```python
from build123d import *

# Parameters (mm, degrees)
EXTRUDE_1_DEPTH          = 22.5
EXTRUDE_2_DEPTH          = 5
EXTRUDE_3_DEPTH          = 4
CUT_EXTRUDE_1_DEPTH      = 23
CUT_EXTRUDE_1_DEPTH_BACK = 8
SKETCH_2_4_R             = 4
CUT_EXTRUDE_2_DEPTH      = 17.5
FILLET_1_R               = 5
SKETCH_4_R               = 4
CUT_EXTRUDE_4_DEPTH      = 35
SKETCH_5_R               = 4
CUT_EXTRUDE_5_DEPTH      = 47
FILLET_2_R               = 10
FILLET_3_R               = 1
CHAMFER_1_SIZE           = 1.6


with BuildPart() as part:
    # Sketch 1 → Extrude 1 (new, symmetric)
    with BuildSketch(Plane.XY):
        Polygon((0, 0), (135, 0), (135, 8), (107, 8), (107, 40), (57, 40), (32, 8), (0, 8), align=None)
    extrude(amount=EXTRUDE_1_DEPTH, both=True)

    # Sketch 2 → Extrude 2 (add, symmetric)
    with BuildSketch(Plane.XY):
        with BuildLine():
            Line((8, 8), (8, 25))
            ThreePointArc((8, 25), (10.343145751, 30.656854249), (16, 33))
            Line((16, 33), (51.53125, 33))
            Line((51.53125, 33), (32, 8))
            Line((32, 8), (8, 8))
        make_face()
    extrude(amount=EXTRUDE_2_DEPTH, both=True)

    # Sketch 2_3 → Extrude 3 (add, symmetric)
    with BuildSketch(Plane.XY):
        Polygon((107, 40), (135, 8), (107, 8), align=None)
    extrude(amount=EXTRUDE_3_DEPTH, both=True)

    # Sketch 2_4 → Cut-Extrude 1 (cut, two sides: drawn at the far end of the back side and taken through both)
    with BuildSketch(Plane.XY.offset(-CUT_EXTRUDE_1_DEPTH_BACK)):
        with Locations((16, 25)):
            Circle(SKETCH_2_4_R)
    extrude(amount=CUT_EXTRUDE_1_DEPTH + CUT_EXTRUDE_1_DEPTH_BACK, mode=Mode.SUBTRACT)

    # Sketch 3 → Cut-Extrude 2 (cut, symmetric)
    with BuildSketch(Plane.XY):
        Polygon((35.901970252, 0), (59.339470252, 30), (91, 30), (91, 0), align=None)
    extrude(amount=CUT_EXTRUDE_2_DEPTH, both=True, mode=Mode.SUBTRACT)

    # Fillet 1
    fillet_1_edges = [part.edges().sort_by_distance(p)[0] for p in [
        (107, 8, 13.25),
        (107, 8, -13.25),
    ]]
    fillet(fillet_1_edges, radius=FILLET_1_R)

    # Sketch 4 → Cut-Extrude 4 (cut)
    with BuildSketch(Plane.XZ):
        with Locations(Location((7.5, 15, 0), (0, 0, 270))):
            Circle(SKETCH_4_R)
        with Locations((7.5, -15)):
            Circle(SKETCH_4_R)
        with Locations((127.5, -15)):
            Circle(SKETCH_4_R)
        with Locations(Location((127.5, 15, 0), (0, 0, 270))):
            Circle(SKETCH_4_R)
    extrude(amount=-CUT_EXTRUDE_4_DEPTH, mode=Mode.SUBTRACT)

    # Sketch 5 → Cut-Extrude 5 (cut)
    with BuildSketch(Plane(origin=(0, 40, 0), x_dir=(1, 0, 0), z_dir=(0, 1, 0))):
        with Locations(Location((98, 0, 0), (0, 0, 180))):
            Circle(SKETCH_5_R)
    extrude(amount=-CUT_EXTRUDE_5_DEPTH, mode=Mode.SUBTRACT)

    # Fillet 2
    fillet_2_edges = [part.edges().sort_by_distance(p)[0] for p in [
        (135, 4, 22.5),
        (0, 4, -22.5),
        (0, 4, 22.5),
        (135, 4, -22.5),
    ]]
    fillet(fillet_2_edges, radius=FILLET_2_R)

    # Fillet 3
    fillet_3_edges = [part.edges().sort_by_distance(p)[0] for p in [
        (41.765625, 20.5, 5),
        (41.765625, 20.5, -5),
        (91, 15, -17.5),
        (91, 30, 0),
        (47.620720252, 15, -17.5),
        (75.169735126, 30, -17.5),
        (59.339470252, 30, 0),
        (91, 15, 17.5),
        (75.169735126, 30, 17.5),
        (47.620720252, 15, 17.5),
    ]]
    fillet(fillet_3_edges, radius=FILLET_3_R)

    # Chamfer 1
    chamfer_1_edges = [part.edges().sort_by_distance(p)[0] for p in [
        (102, 40, 0),
    ]]
    chamfer(chamfer_1_edges, length=CHAMFER_1_SIZE)


solid = part.part
```
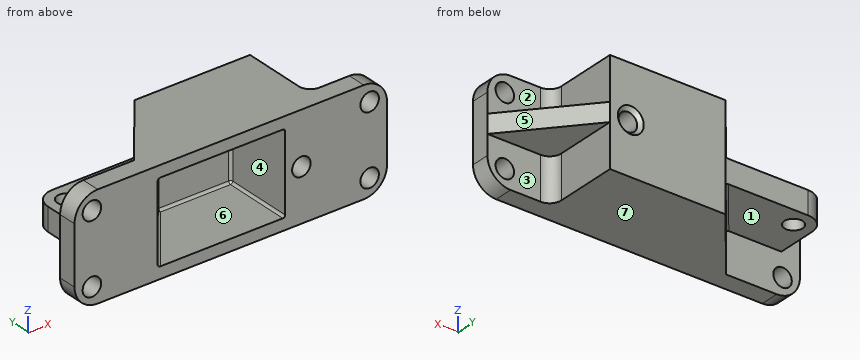
Can you work these out from the model? Positions are in its coordinate system, mm. Face numbers are marked on the shaded views. A direction names the side the tool comes from. Give positions to 0.01 mm unless a question says otherwise; leave off trailing zeros. Loops run counter-clockwise (first coordinate to the right, second up) from the corner with the lowest first, then second, coordinate; pieces in that order, holes last. Notation, with made-up numbers: M 59,18.25 L 118,18.25 A24 cw 118,56.25 Z; hole C 4.5,43 d5. An arc over 180 degrees is marked long. One line per item, written item: value.
(1) I need wall thicknesses on line 1 (Z direction, x = 56.5, y = 24); line 2 (X direction, y = 3, z = 15); line 3 (X direction, y = 25, z = -1) (3 decimals). Which ranges of each line are inside material? Lowest first, please.
Returned:
line 1: -22.5 to -17.5, 17.5 to 22.5
line 2: 0.32 to 3.5, 11.5 to 38.25, 91 to 123.5, 131.5 to 134.68
line 3: 8 to 12, 20 to 55.433, 91 to 94.127, 101.873 to 120.125
(2) Suppose I cut it at A-A on z = 0. List the corners of the cut face in (x, y) for me.
Returned:
outline: M 0,0 L 35.9,0 L 59.04,29.62 A1 cw 59.83,30 L 90,30 A1 cw 91,29 L 91,0 L 94,0 L 94,38.4 L 92.4,40 L 57,40 L 51.53,33 L 16,33 A8 ccw 8,25 L 8,8 L 0,8 Z; M 102,0 L 135,0 L 135,8 L 107,40 L 103.6,40 L 102,38.4 Z; hole C 16,25 d8
(3) Will these pins go through, and if not, where does the flat tip stop? pin 1 (15 mm diameter, centred on x = 82.5, z = 8, fed in from -Y); pin 2 (14 mm diameter, centred on x = 117.5, y = 30, fed in from +Z); pin 3 (8 mm diameter, centred on x = 23, y = 25.5, fed in from +Z).
Returned:
pin 1: y = 30
pin 2: z = 4
pin 3: z = 5
(4) Suppose I cut it at D-D on y = 36. List the corners of the cut face in (x, z) for me (3 decimals), plus the area to 3 significant figures.
Returned:
outline: M 53.875,-22.5 L 107,-22.5 L 107,-4 L 110.5,-4 L 110.5,4 L 107,4 L 107,22.5 L 53.875,22.5 Z; hole C 98,0 d8
area: 2,370 mm^2
(5) We'd pull the mould along Z, two halves only. Please class the marked faces 5, 6 and 7: released by +Z, released by -Z, zero draft, split by the parting line, or undercut.
Returned:
face 5: zero draft
face 6: undercut
face 7: released by -Z
(6) Which directions (+Z, -Z, +X, -X, +Y, -Y) give clear straight access to the entire face, cutting with the end or side of a thin tool? Please do the marked faces 1, 2, 3 and 4.
Returned:
face 1: -Z, -X, +Y
face 2: +Z, +X, +Y
face 3: -Z, +X, +Y
face 4: -Y
(7) Suppose I cut it at B-B on z = -15. List the corners of the cut face in (x, y) for me.
Returned:
outline: M 0.32,0 L 3.5,0 L 3.5,8 L 0.32,8 Z; M 11.5,0 L 35.9,0 L 59.04,29.62 A1 cw 59.83,30 L 90,30 A1 cw 91,29 L 91,0 L 123.5,0 L 123.5,8 L 112,8 A5 cw 107,13 L 107,40 L 57,40 L 32,8 L 11.5,8 Z; M 131.5,0 L 134.68,0 L 134.68,8 L 131.5,8 Z
(8) Suppose I cut it at C-C on x = 127.5. List the corners of the cut face in (y, z) for me.
Returned:
outline: M 0,-22.18 L 8,-22.18 L 8,-19 L 0,-19 Z; M 0,-11 L 8,-11 L 8,-4 L 16.57,-4 L 16.57,4 L 8,4 L 8,11 L 0,11 Z; M 0,19 L 8,19 L 8,22.18 L 0,22.18 Z
